from build123d import *

# Parameters (mm, degrees)
BOSS_EXTRUDE1_DEPTH             = 450
CUT_EXTRUDE1_DEPTH              = 320.536163525
CUT_EXTRUDE1_DEPTH_BACK         = 87.9500001
BOSS_EXTRUDE2_REACH             = 321.536
BOSS_EXTRUDE2_DIRECTION_2_REACH = 88.95
SKETCH4_W                       = 40
SKETCH4_H                       = 10
BOSS_EXTRUDE3_DEPTH             = 50


with BuildPart() as part:
    # Sketch1 → Boss-Extrude1 (new body)
    with BuildSketch(Plane.XY):
        with BuildLine():
            Line((0, 0), (0, -86.95))
            Line((0, -86.95), (90, -86.95))
            Line((90, -86.95), (90, 163.05))
            add(Edge.make_bspline(
                [(90, 163.05), (72.317416943, 256.499426115), (1.7e-06, 319.536163425)],
                knots=[0, 0, 0, 1, 1, 1], degree=2))
            Line((1.7e-06, 319.536163425), (-1.971240178, 317.274702513))
            add(Edge.make_bspline(
                [(87, 162.76796294), (86.63530579, 164.685544789), (85.866737034, 168.522541651), (84.193801862, 176.09415534), (81.838470508, 185.417428941), (78.592614297, 196.364076295), (73.704594381, 210.644362496), (66.544776494, 227.902696365), (56.272326819, 247.671791898), (44.316806262, 266.505130738), (32.948415938, 281.423453125), (23.007866651, 292.89431167), (15.129804099, 301.265055213), (8.209142943, 308.04969842), (2.465529724, 313.357146881), (-0.486511784, 315.980513091), (-1.971240178, 317.274702513)],
                knots=[0.001490309, 0.001490309, 0.001490309, 0.001490309, 0.032693737, 0.063897165, 0.12630402, 0.188710876, 0.251117732, 0.375931443, 0.500745154, 0.625558866, 0.750372577, 0.812779433, 0.875186289, 0.937593144, 0.968796572, 1, 1, 1, 1], degree=3))
            Line((87, 162.76796294), (87, -83.95))
            Line((87, -83.95), (3, -83.95))
            Line((3, -83.95), (3, 0))
            Line((3, 0), (0, 0))
        make_face()
    extrude(amount=BOSS_EXTRUDE1_DEPTH)

    # Sketch2 → Cut-Extrude1 (cut, two sides)
    with BuildSketch(Plane(origin=(0, 0, 0), x_dir=(1, 0, 0), z_dir=(0, 1, 0))) as cut_extrude1_sk:
        Polygon((-1.971240178, -450), (90, -400), (90, -450), align=None)
        Polygon((90, 0), (90, -50), (-1.971240178, 0), align=None)
    extrude(amount=CUT_EXTRUDE1_DEPTH, mode=Mode.SUBTRACT)
    extrude(cut_extrude1_sk.sketch, amount=-CUT_EXTRUDE1_DEPTH_BACK, mode=Mode.SUBTRACT)

    # Sketch3 → Boss-Extrude2 (add, up to next)
    with BuildSketch(Plane(origin=(0, 0, 0), x_dir=(1, 0, 0), z_dir=(0, 1, 0)), mode=Mode.PRIVATE) as boss_extrude2_sk1:
        Polygon((-1.971240178, -446), (90, -396), (90, -400), (-1.971240178, -450), align=None)
    boss_extrude2_tool1 = extrude(boss_extrude2_sk1.sketch, amount=BOSS_EXTRUDE2_REACH, mode=Mode.PRIVATE) - part.part
    add(boss_extrude2_tool1.solids().sort_by_distance((44.01438, 0, 423))[0])
    # Sketch3 → Boss-Extrude2 (add, up to next)
    with BuildSketch(Plane(origin=(0, 0, 0), x_dir=(1, 0, 0), z_dir=(0, 1, 0)), mode=Mode.PRIVATE) as boss_extrude2_sk2:
        Polygon((-1.971240178, -4), (-1.971240178, 0), (90, -50), (90, -54), align=None)
    boss_extrude2_tool2 = extrude(boss_extrude2_sk2.sketch, amount=BOSS_EXTRUDE2_REACH, mode=Mode.PRIVATE) - part.part
    add(boss_extrude2_tool2.solids().sort_by_distance((44.01438, 0, 27))[0])

    # Sketch3 → Boss-Extrude2 direction 2 (add, up to next)
    with BuildSketch(Plane(origin=(0, 0, 0), x_dir=(1, 0, 0), z_dir=(0, 1, 0)), mode=Mode.PRIVATE) as boss_extrude2_direction_2_sk1:
        Polygon((-1.971240178, -446), (90, -396), (90, -400), (-1.971240178, -450), align=None)
    boss_extrude2_direction_2_tool1 = extrude(boss_extrude2_direction_2_sk1.sketch, amount=-BOSS_EXTRUDE2_DIRECTION_2_REACH, mode=Mode.PRIVATE) - part.part
    add(boss_extrude2_direction_2_tool1.solids().sort_by_distance((44.01438, 0, 423))[0])
    # Sketch3 → Boss-Extrude2 direction 2 (add, up to next)
    with BuildSketch(Plane(origin=(0, 0, 0), x_dir=(1, 0, 0), z_dir=(0, 1, 0)), mode=Mode.PRIVATE) as boss_extrude2_direction_2_sk2:
        Polygon((-1.971240178, -4), (-1.971240178, 0), (90, -50), (90, -54), align=None)
    boss_extrude2_direction_2_tool2 = extrude(boss_extrude2_direction_2_sk2.sketch, amount=-BOSS_EXTRUDE2_DIRECTION_2_REACH, mode=Mode.PRIVATE) - part.part
    add(boss_extrude2_direction_2_tool2.solids().sort_by_distance((44.01438, 0, 27))[0])

    # Sketch4 → Boss-Extrude3 (add)
    with BuildSketch(Plane(origin=(90, 0, 0), x_dir=(0, 0, -1), z_dir=(1, 0, 0))):
        with Locations((-295, 25)):
            Rectangle(SKETCH4_W, SKETCH4_H)
        with Locations((-155, 45)):
            Rectangle(SKETCH4_W, SKETCH4_H)
        with Locations((-155, 25)):
            Rectangle(SKETCH4_W, SKETCH4_H)
        with Locations((-295, 45)):
            Rectangle(SKETCH4_W, SKETCH4_H)
    extrude(amount=BOSS_EXTRUDE3_DEPTH)


solid = part.part
Build history of the part. All positions in model axes, mm. A direction names the side the tool comes from. Coordinates: 2 decimals unless noted, no trailing zeros. Order: outer loops, then holes, each group sorted by start corner. A loop starts at its lowest first (then second) coordinate and runs counter-clockwise, first axis right, second up. Notation, with made-up numbers: (-2.75, 17) -> (47.25, 17) arc R17 ccw to (47.25, 31) -> close; hole circle Ø6 at (-14.75, 30). An arc over 180 degrees is marked (long way). One line per item, written item: value.
(1) Slice it at B-B, the plane y = 14. List the corners of the cut face in (x, z).
Checked values:
outline: (-1.97, 0) -> (90, 50) -> (90, 400) -> (-1.97, 450) -> (-1.97, 446) -> (87, 397.63) -> (87, 52.37) -> (-1.97, 4) -> close
(2) Drop flat-ended pins along their axis: pin 1 Ø5 at (x, y) = (118.5, 24) entering from +Z; pin 2 Ø10 at (x, y) = (53.5, 210) entering from +Z; pin 3 Ø3 at (x, y) = (123, 22.5) entering from -Z. Give the stop position or say it passes through.
Checked values:
pin 1: z = 315
pin 2: z = 422.56
pin 3: z = 135
(3) Tool access for faces 1 (the flat face through (3, -43, 222)), 2 (the flat face through (115, 30, 155)), 3 (the flat face through (115, 25, 275)): list every direction of +Z, -Z, +X, -X, +Y, -Y with a clear straight run to the whole face (end or side of a thin tool).
Checked values:
face 1: none
face 2: +Z, -Z, +X
face 3: +X, +Y, -Y
(4) Probe line 1 (X direction, y = -40, z = 356); line 2 (Y direction, x = 104.5, z = 282.5); line 3 (X direction, y = 104, z = 162). List the from-to ranges inside material, lowest first. Write a range as [from, to].
Checked values:
line 1: [0, 3], [87, 90]
line 2: [20, 30], [40, 50]
line 3: [87, 90]
(5) Slice it at A-A, the plane x = 127.5. List the corners of the cut face in (y, z), plus the area to 3 significant figures.
Checked values:
outline: (20, 135) -> (30, 135) -> (30, 175) -> (20, 175) -> close; (20, 275) -> (30, 275) -> (30, 315) -> (20, 315) -> close; (40, 135) -> (50, 135) -> (50, 175) -> (40, 175) -> close; (40, 275) -> (50, 275) -> (50, 315) -> (40, 315) -> close
area: 1,600 mm2
(6) Mould opens along Y. For faces 4 (the flat face through (115, 45, 135)), 5 (the flat face through (115, 50, 155)), 6 (the flat face through (115, 20, 155)), 7 (the flat face through (87, 41, 223)) say: pulls with the +Y half, pulls with the -Y half, needs draft (parallel to the pull), parting line crosses it, or undercut.
Checked values:
face 4: needs draft
face 5: pulls with the +Y half
face 6: pulls with the -Y half
face 7: undercut
